Read the model definition and answer for the solid it produces. Units are mm, in the model's axes. A direction names the side the tool comes from. Coordinates: 2 decimals unless noted, no trailing zeros. Loops run counter-clockwise (first coordinate to the right, second up) from the corner with the lowest first, then second, coordinate; pieces in that order, holes last.
Autodesk Inventor part; units mm, degrees
ref_plane "YZ Plane" through (0, 0, 0) normal (1, 0, 0) x (0, 1, 0)
ref_plane "XZ Plane" through (0, 0, 0) normal (0, 1, 0) x (-1, 0, 0)
ref_plane "XY Plane" through (0, 0, 0) normal (0, 0, 1) x (1, 0, 0)
sketch "Sketch1" plane through (0, 0, 0) normal (0, 0, 1) x (1, 0, 0)
  line L0 (-12.7, 28.8544) -> (-28.8544, 28.8544)
  line L1 (-28.8544, 28.8544) -> (-31.75, 28.8544)
  line L2 (-31.75, 28.8544) -> (-31.75, 12.7)
  line L3 (-31.75, 12.7) -> (-28.8544, 12.7)
  line L4 (-28.8544, 12.7) -> (-28.8544, -12.7)
  line L5 (-28.8544, -12.7) -> (-31.75, -12.7)
  line L6 (-31.75, -12.7) -> (-31.75, -28.8544)
  line L7 (-31.75, -28.8544) -> (-28.8544, -28.8544)
  line L8 (-28.8544, -28.8544) -> (-12.7, -28.8544)
  line L9 (-12.7, -28.8544) -> (-12.7, -31.75)
  line L10 (-12.7, -31.75) -> (12.7, -31.75)
  line L11 (12.7, -31.75) -> (12.7, -28.8544)
  line L12 (12.7, -28.8544) -> (28.8544, -28.8544)
  line L13 (28.8544, -28.8544) -> (31.75, -28.8544)
  line L14 (31.75, -28.8544) -> (31.75, -12.7)
  line L15 (31.75, -12.7) -> (28.8544, -12.7)
  line L16 (28.8544, -12.7) -> (28.8544, 12.7)
  line L17 (28.8544, 12.7) -> (31.75, 12.7)
  line L18 (31.75, 12.7) -> (31.75, 28.8544)
  line L19 (31.75, 28.8544) -> (28.8544, 28.8544)
  line L20 (28.8544, 28.8544) -> (12.7, 28.8544)
  line L21 (12.7, 28.8544) -> (12.7, 31.75)
  line L22 (12.7, 31.75) -> (-12.7, 31.75)
  line L23 (-12.7, 31.75) -> (-12.7, 28.8544)
  point P0 (0, 0)
extrude "Extrusion1" add sketch "Sketch1" along normal blind 2.8956
properties part number "inside_box_left_right" material "Polycarbonate, Clear"
Item 1: Find the intervals of material crossed by line 1 along X through (y, z) = (9, 0.9), in increasing order.
Numbers:
line 1: x = -28.85 to 28.85
Item 2: Given pin 1 (0.9 mm diameter, centred on x = -31, z = 1, fed in from +Y); pin 2 (0.9 mm diameter, centred on y = 30.5, z = 1, fed in from -X); pin 3 (1.4 mm diameter, centred on x = 30.5, z = 1.5, fed in from -Y), each flat-ended and moving along its own axis, determine where each tip first touches the part or whether it passes through.
Numbers:
pin 1: stops at y = 28.85
pin 2: stops at x = -12.7
pin 3: stops at y = -28.85
Item 3: Which of the six approach directions +Z, -Z, +X, -X, +Y, -Y give full straight-line access (tool end or side, diameter ignored) to faces 1 (the face through (-30, -12.7, 1)), 2 (the face through (-12.7, 30, 1)), 3 (the face through (12.7, 30, 1))?
Numbers:
face 1: +Z, -Z, -X
face 2: +Z, -Z, -X, +Y
face 3: +Z, -Z, +X, +Y
Item 4: A cutting plane is placed at A-A on z = 1.6. Determine the outline of the cut face in (x, y).
Numbers:
outline: (-31.75, -28.85) - (-12.7, -28.85) - (-12.7, -31.75) - (12.7, -31.75) - (12.7, -28.85) - (31.75, -28.85) - (31.75, -12.7) - (28.85, -12.7) - (28.85, 12.7) - (31.75, 12.7) - (31.75, 28.85) - (12.7, 28.85) - (12.7, 31.75) - (-12.7, 31.75) - (-12.7, 28.85) - (-31.75, 28.85) - (-31.75, 12.7) - (-28.85, 12.7) - (-28.85, -12.7) - (-31.75, -12.7) - close
Item 5: Determine the mould class of faces 4 (the face through (0, 31.75, 1)), 5 (the face through (30, -12.7, 1)), 6 (the face through (0, -31.75, 1)) for opening direction Y: released by +Y, released by -Y, zero draft, split by the parting line, or undercut.
Numbers:
face 4: released by +Y
face 5: undercut
face 6: released by -Y
Item 6: A cutting plane is placed at B-B on x = 17.5. Determine the outline of the cut face in (y, z), then the cut area to 3 significant figures.
Numbers:
outline: (-28.85, 0) - (28.85, 0) - (28.85, 2.9) - (-28.85, 2.9) - close
area: 167 mm2
